The listing builds one solid part. Answer for the finished solid, in the listing's coordinates (mm). A direction names the side the tool comes from. Give positions to 0.01 mm unless a question says otherwise; leave off trailing zeros. Write each loop counter-clockwise with the first axis right and the second up, starting at its lowest first coordinate (ties: lowest second). Pieces come first, ordered by that corner, then holes. Notation, with made-up numbers: M 66,-33.5 L 77,-33.5 A24 ccw 77,-2.5 Z; hole C -26,44 d9. An arc over 180 degrees is marked long. Return JSON: item names as keys, results as strings.
from build123d import *

# Parameters (mm, degrees)
SKETCH1_R           = 12.5
BOSS_EXTRUDE2_DEPTH = 15
SKETCH2_R           = 14
BOSS_EXTRUDE3_DEPTH = 0.5
SKETCH3_R           = 12.25
CUT_EXTRUDE1_DEPTH  = 14.5
FILLET1_R           = 2.5
FILLET2_R           = 2.5


with BuildPart() as part:
    # Sketch1 → Boss-Extrude2 (new body)
    with BuildSketch(Plane(origin=(0, 0, 0), x_dir=(1, 0, 0), z_dir=(0, 1, 0))):
        with Locations(Location((0, 0, 0), (0, 0, 270))):
            Circle(SKETCH1_R)
    extrude(amount=BOSS_EXTRUDE2_DEPTH)

    # Sketch2 → Boss-Extrude3 (add)
    with BuildSketch(Plane(origin=(0, 0, 0), x_dir=(1, 0, 0), z_dir=(0, 1, 0))):
        with Locations(Location((0, 0, 0), (0, 0, 270))):
            Circle(SKETCH2_R)
    extrude(amount=BOSS_EXTRUDE3_DEPTH)

    # Sketch3 → Cut-Extrude1 (cut)
    with BuildSketch(Plane(origin=(0, 0, 0), x_dir=(1, 0, 0), z_dir=(0, 1, 0))):
        with Locations(Location((0, 0, 0), (0, 0, 90))):
            Circle(SKETCH3_R)
    extrude(amount=CUT_EXTRUDE1_DEPTH, mode=Mode.SUBTRACT)

    # Fillet1
    fillet1_edges = [part.edges().sort_by_distance(p)[0] for p in [
        (0, 15, -12.5),
    ]]
    fillet(fillet1_edges, radius=FILLET1_R)

    # Fillet2
    fillet2_edges = [part.edges().sort_by_distance(p)[0] for p in [
        (0, 14.5, 12.25),
    ]]
    fillet(fillet2_edges, radius=FILLET2_R)


solid = part.part
Item 1: A cutting plane is placed at B-B, the plane x = 0. Write down the section's boundary in (y, z).
Geometry results:
{"outline": "M 0,-14 L 0.5,-14 L 0.5,-12.5 L 12.5,-12.5 A2.5 ccw 15,-10 L 15,10 A2.5 ccw 12.5,12.5 L 0.5,12.5 L 0.5,14 L 0,14 L 0,12.25 L 12,12.25 A2.5 cw 14.5,9.75 L 14.5,-9.75 A2.5 cw 12,-12.25 L 0,-12.25 Z"}
Item 2: Find the intervals of material crossed by line 1 (X direction, y = 6.5, z = 0); line 2 (X direction, y = 14, z = -5); line 3 (Y direction, x = -2.5, z = -7.75), in increasing order.
Geometry results:
{"line 1": "x = -12.5 to -12.25, 12.25 to 12.5", "line 2": "x = -10.91 to -10.08, 10.08 to 10.91", "line 3": "y = 14.5 to 15"}
Item 3: Determine the mould class of faces 1 (the cylindrical face through (-13.67, 0.25, -3.03)), 2 (the flat face through (0, 14.5, 0)), 3 (the flat face through (0, 15, 0)) for opening direction X: +X half, -X half, draft (parallel to the pull), parting line (faces both ways), or undercut.
Geometry results:
{"face 1": "parting line", "face 2": "undercut", "face 3": "draft"}
Item 4: A cutting plane is placed at A-A, the plane z = 0. Write down the section's boundary in (x, y).
Geometry results:
{"outline": "M -14,0 L -12.25,0 L -12.25,12 A2.5 cw -9.75,14.5 L 9.75,14.5 A2.5 cw 12.25,12 L 12.25,0 L 14,0 L 14,0.5 L 12.5,0.5 L 12.5,12.5 A2.5 ccw 10,15 L -10,15 A2.5 ccw -12.5,12.5 L -12.5,0.5 L -14,0.5 Z"}
Item 5: Which of the six approach directions +Z, -Z, +X, -X, +Y, -Y give full straight-line access (tool end or side, diameter ignored) to faces 4 (the flat face through (11.5, 0.5, -5.3)), 5 (the flat face through (-12.4, 0, -0.1)), 6 (the cylindrical face through (-3.68, 5.916, -11.684))?
Geometry results:
{"face 4": "+Y", "face 5": "+Z, -Z, +X, -X, -Y", "face 6": "-Y"}
Item 6: A cutting plane is placed at C-C, the plane y = 13. Write down the section's boundary in (x, z), plus the area to 3 significant figures.
Geometry results:
{"outline": "C 0,0 d24.9; hole C 0,0 d24.08", "area": "31.4 mm2"}
Item 7: Given pin 1 Ø12 at (x, z) = (1, 4.5) entering from -Y; pin 2 Ø6 at (x, y) = (5.5, 4) entering from -Z; pin 3 Ø6 at (y, z) = (1.5, 4) entering from +X, each flat-ended and moving along its own axis, determine where each tip first touches the part or whether it passes through.
Geometry results:
{"pin 1": "stops at y = 14.35", "pin 2": "stops at z = -12.25", "pin 3": "stops at x = 13.95"}
